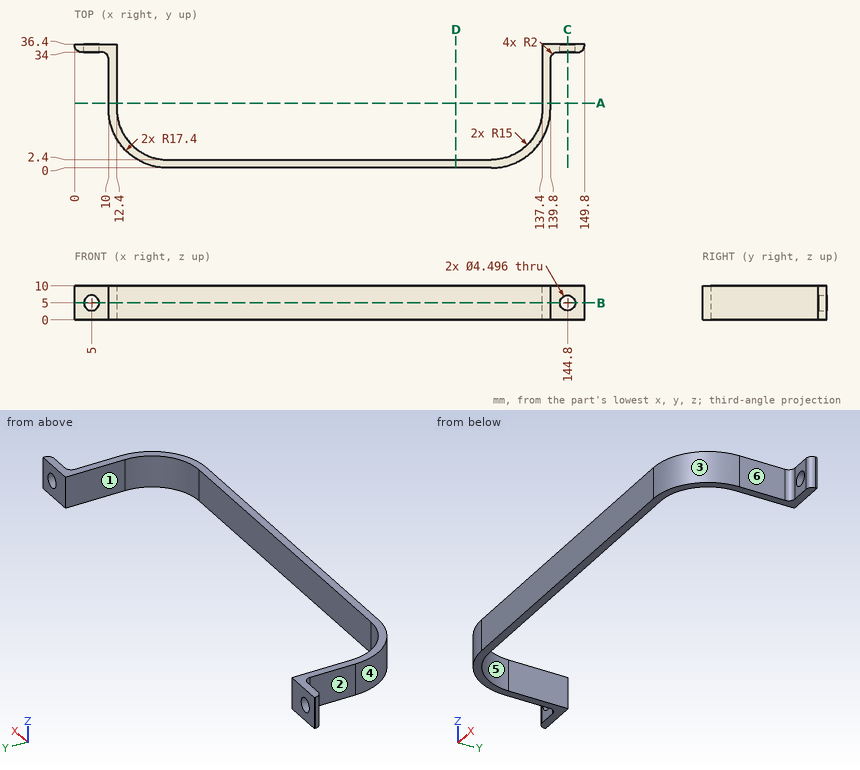
Design review of the part shown in the three views and the two pictorial views. Dimensions are in mm from the part's minimum x, y and z. A direction names the side the tool comes from. Round coordinates to 2 decimals unless told otherwise and drop trailing zeros. Loops run counter-clockwise (first coordinate to the right, second up) from the corner with the lowest first, then second, coordinate; pieces in that order, holes last.
(1) We need section B-B (z = 5). Give the boundary of the cut face in (x, y).
Returned:
outline: (0, 36) arc R2 ccw to (2, 34) - (2.75, 34) - (2.75, 36.4) - (0, 36.4) - close; (7.25, 34) - (8, 34) arc R2 cw to (10, 32) - (10, 17.4) arc R17.4 ccw to (27.4, 0) - (122.4, 0) arc R17.4 ccw to (139.8, 17.4) - (139.8, 32) arc R2 cw to (141.8, 34) - (142.55, 34) - (142.55, 36.4) - (137.4, 36.4) - (137.4, 17.4) arc R15 cw to (122.4, 2.4) - (27.4, 2.4) arc R15 cw to (12.4, 17.4) - (12.4, 36.4) - (7.25, 36.4) - close; (147.05, 34) - (147.8, 34) arc R2 ccw to (149.8, 36) - (149.8, 36.4) - (147.05, 36.4) - close
(2) We need section C-C (x = 144.8). Give the boundary of the cut face in (y, z), plus the area to 3 significant figures.
Returned:
outline: (34, 0) - (36.4, 0) - (36.4, 2.75) - (34, 2.75) - close; (34, 7.25) - (36.4, 7.25) - (36.4, 10) - (34, 10) - close
area: 13.2 mm2
(3) Clearance check with flat-ended pins moving along their axes: P1, Ø2, axis at y = 26, z = 1, coming from the -X side; P2, Ø1, axis at y = 24.5, z = 4, coming from the +X side; P3, Ø6, axis at y = 12, z = 7, coming from the +X side. State where each tip first meets the part, or that it passes through.
Returned:
P1: stops at x = 10
P2: stops at x = 139.8
P3: stops at x = 139.63
(4) Mouldability with a two-part tool opening along X and no side actions: class the marked faces 4, 5 and 6 as released by +X, released by -X, zero draft, split by the parting line, or undercut.
Returned:
face 4: released by -X
face 5: undercut
face 6: released by +X
(5) We need section D-D (x = 112). Give the boundary of the cut face in (y, z), plus the area to 3 significant figures.
Returned:
outline: (0, 0) - (2.4, 0) - (2.4, 10) - (0, 10) - close
area: 24.0 mm2
(6) Tool access review of the marked faces 1, 2 and 3: name each direction out of +Z, -Z, +X, -X, +Y, -Y from which nothing blocks a thin tool from reaching the whole face with its end or side.
Returned:
face 1: +Z, -Z, +Y
face 2: +Z, -Z, -X, -Y
face 3: +Z, -Z, +X, -Y
(7) We need section A-A (y = 19). Give the boundary of the cut face in (x, z).
Returned:
outline: (10, 0) - (12.4, 0) - (12.4, 10) - (10, 10) - close; (137.4, 0) - (139.8, 0) - (139.8, 10) - (137.4, 10) - close
(8) Wall thickness on line 1 along Z through (x, y) = (5, 35.3); line 2 along X through (y, z) = (23, 4.5); line 3 along X through (y, z) = (9.5, 5.75): over which ranges is each line inside the solid? List them lowest first.
Returned:
line 1: z = 0 to 2.75, 7.25 to 10
line 2: x = 10 to 12.4, 137.4 to 139.8
line 3: x = 11.9 to 14.65, 135.15 to 137.9
